Work out the finished part from the listing and answer in its coordinate system (mm). Face numbers are marked on the shaded views. A direction names the side the tool comes from. Round coordinates to 2 decimals unless told otherwise and drop trailing zeros. Write each loop counter-clockwise with the first axis right and the second up, starting at its lowest first coordinate (ties: lowest second). Pieces come first, ordered by that corner, then holes. Notation, with made-up numbers: M 31,7.5 L 36,7.5 A23 cw 36,16.5 Z; hole C 53.25,-0.5 d7. An arc over 180 degrees is marked long. Answer in a Markdown table with one row per item.
```python
from build123d import *

# Parameters (mm, degrees)
SKETCH1_R           = 6.35
BOSS_EXTRUDE1_DEPTH = 10.16
DOME1_FACE_RADIUS   = 6.35
DOME1_HEIGHT        = 2.54
SKETCH3_W           = 3.81
SKETCH3_H           = 3.81
CUT_EXTRUDE1_DEPTH  = 7.62
SKETCH5_W           = 4.7625
SKETCH5_H           = 4.7625
BOSS_EXTRUDE2_DEPTH = 12.7
SKETCH6_R           = 1.5875
CUT_EXTRUDE2_DEPTH  = 12.7


with BuildPart() as part:
    # Sketch1 → Boss-Extrude1 (new body)
    with BuildSketch(Plane.XY):
        Circle(SKETCH1_R)
    extrude(amount=BOSS_EXTRUDE1_DEPTH)

    # Dome1: a dome of height H over a round flat face of radius A is a cap of a sphere of radius (A * A + H * H) / (2 * H)
    dome1_r = (DOME1_FACE_RADIUS * DOME1_FACE_RADIUS + DOME1_HEIGHT * DOME1_HEIGHT) / (2 * DOME1_HEIGHT)
    dome1_base = Plane((0, 0, 10.16), z_dir=(0, 0, 1))
    with Locations(dome1_base.offset(DOME1_HEIGHT - dome1_r)):
        dome1_ball = Sphere(dome1_r, mode=Mode.PRIVATE)
    add(split(dome1_ball, bisect_by=dome1_base, keep=Keep.TOP, mode=Mode.PRIVATE))

    # Sketch3 → Cut-Extrude1 (cut)
    with BuildSketch(Plane(origin=(0, 0, 7.62), x_dir=(-1, 0, 0), z_dir=(0, 0, -1))):
        Rectangle(SKETCH3_W, SKETCH3_H)
    extrude(amount=CUT_EXTRUDE1_DEPTH, mode=Mode.SUBTRACT)

    # Sketch5 → Boss-Extrude2 (add)
    with BuildSketch(Plane(origin=(0, 0, 7.62), x_dir=(-1, 0, 0), z_dir=(0, 0, -1))):
        Rectangle(SKETCH5_W, SKETCH5_H)
    extrude(amount=-BOSS_EXTRUDE2_DEPTH)

    # Sketch6 → Cut-Extrude2 (cut)
    with BuildSketch(Plane(origin=(-1.905, 0, 0), x_dir=(0, 0, -1), z_dir=(1, 0, 0))):
        with Locations((-3.96875, 0)):
            Circle(SKETCH6_R)
    extrude(amount=-CUT_EXTRUDE2_DEPTH, mode=Mode.SUBTRACT)


solid = part.part
```
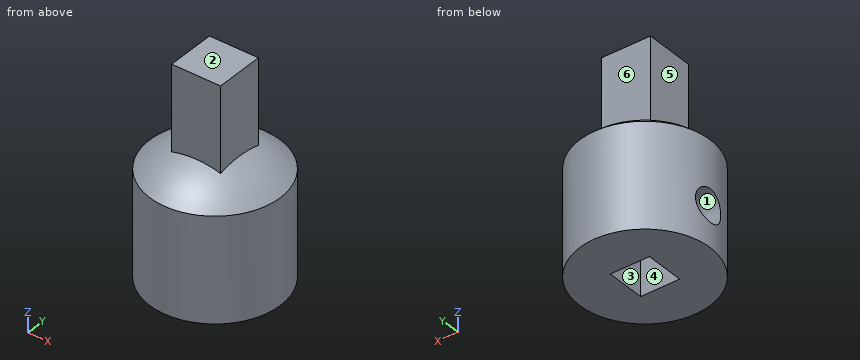
1. The part is cut by section C-C (z = 4). Determine the outline of the cut face in (x, y) (3 decimals), plus the area to 3 significant figures.
Calculated:
| item | result |
|---|---|
| outline | M -6.148,-1.587 A6.35 ccw long -6.148,1.587 L -1.905,1.587 L -1.905,1.905 L 1.905,1.905 L 1.905,-1.905 L -1.905,-1.905 L -1.905,-1.587 Z |
| area | 98.3 mm² |
2. The part is cut by section D-D (y = -4.5). Determine the outline of the cut face in (x, z).
Calculated:
| item | result |
|---|---|
| outline | M -4.48,0 L 4.48,0 L 4.48,10.16 A8.03 ccw -4.48,10.16 Z |
3. A tool of negligible diameter and unlimited length cuts with its end or side. For the marked faces 1 and 2, from which of +Z, -Z, +X, -X, +Y, -Y can it reach the whole face along a straight path? Write none if from no direction.
Calculated:
| item | result |
|---|---|
| face 1 | -X |
| face 2 | +Z, +X, -X, +Y, -Y |
4. Determine the mould class of the marked faces 3, 4, 5 and 6 for opening direction Y: released by +Y, released by -Y, zero draft, split by the parting line, or undercut.
Calculated:
| item | result |
|---|---|
| face 3 | undercut |
| face 4 | undercut |
| face 5 | zero draft |
| face 6 | released by +Y |
5. Given pin 1 (5 mm diameter, centred on y = 4.5, z = 16, fed in from +X); pin 2 (3 mm diameter, centred on x = -0.5, y = -1, fed in from -Z); pin 3 (1 mm diameter, centred on y = -1, z = 3, fed in from +X); pin 4 (5 mm diameter, centred on y = -5, z = 10.5, fed in from -X), each flat-ended and moving along its own axis, determine where each tip first touches the part or whether it passes through.
Calculated:
| item | result |
|---|---|
| pin 1 | stops at x = 2.38 |
| pin 2 | stops at z = 0 |
| pin 3 | stops at x = 6.33 |
| pin 4 | stops at x = -5.83 |
6. Consider line 1 along Y through (x, z) = (1, 1.25) (3 decimals); line 2 along Z through (x, y) = (-3.4, 0); line 3 along Y through (x, z) = (1.5, 18.5). Determine where each line is inside the solid, lowest interval first. Write a range as from..to.
Calculated:
| item | result |
|---|---|
| line 1 | y = -6.271..-1.905, 1.905..6.271 |
| line 2 | z = 0..2.38, 5.56..12.05 |
| line 3 | y = -2.38..2.38 |
